```python
from build123d import *

# Parameters (mm, degrees)
F0_R     = 1.5875
F0_W     = 0.381
F0_H     = 9.906
F1_DEPTH = 127
F2_W     = 0.381
F2_H     = 9.906
F3_DEPTH = 127
F7_DEPTH = 127
F5_W     = 1.27
F5_H     = 3.81
F8_DEPTH = 3.175


with BuildPart() as f1:
    # F0 (on Front) → F1 (new body, symmetric)
    with BuildSketch(Plane.XZ):
        Polygon((-8.89, 2.921), (-8.89, -2.921), (-1.4605, -2.921), (-1.0795, -2.921), (1.0795, -2.921), (1.4605, -2.921), (8.89, -2.921), (8.89, 2.921), (3.048, 2.921), (3.048, 9.271), (-3.048, 9.271), (-3.048, 2.921), align=None)
        with Locations((-5.715, 0)):
            Circle(F0_R, mode=Mode.SUBTRACT)
        with Locations((5.715, 0)):
            Circle(F0_R, mode=Mode.SUBTRACT)
        with Locations((-1.27, -7.874)):
            Rectangle(F0_W, F0_H)
        with Locations((1.27, -7.874)):
            Rectangle(F0_W, F0_H)
    extrude(amount=F1_DEPTH, both=True)

    # F2 (on Right) → F3 (intersect, symmetric)
    with BuildSketch(Plane.YZ):
        Polygon((-8.89, 9.271), (-12.954, 9.271), (-12.954, -2.921), (-11.7475, -2.921), (-11.3665, -2.921), (-1.5875, -2.921), (-1.2065, -2.921), (0, -2.921), (0, 9.271), (-3.81, 9.271), (-3.81, 0.1778), (-8.89, 0.1778), align=None)
        with Locations((-1.397, -7.874)):
            Rectangle(F2_W, F2_H)
        with Locations((-11.557, -7.874)):
            Rectangle(F2_W, F2_H)
    extrude(amount=F3_DEPTH, both=True, mode=Mode.INTERSECT)

    # F6 (on Top) → F7 (intersect, symmetric)
    with BuildSketch(Plane.XY):
        Polygon((8.89, 0), (-8.89, 0), (-8.89, -1.905), (-3.048, -1.905), (-3.048, -12.954), (3.048, -12.954), (3.048, -1.905), (8.89, -1.905), align=None)
    extrude(amount=F7_DEPTH, both=True, mode=Mode.INTERSECT)

    # F5 (on plane+point) → F8 (cut, symmetric)
    with BuildSketch(Plane.XZ.offset(6.477)):
        with Locations((0, 7.366)):
            Rectangle(F5_W, F5_H)
    extrude(amount=F8_DEPTH, both=True, mode=Mode.SUBTRACT)


solid = f1.part
```
Could you check a few things on this model? Use its own coordinates, in mm. A direction names the side the tool comes from. Coordinates: 2 decimals unless noted, no trailing zeros. Write each loop counter-clockwise with the first axis right and the second up, starting at its lowest first coordinate (ties: lowest second). Pieces come first, ordered by that corner, then holes. Notation, with made-up numbers: (17, -21.75) -> (31, -21.75) arc R21 ccw to (31, 0.25) -> close; hole circle Ø7 at (12.5, -40). An arc over 180 degrees is marked (long way). One line per question, with ' | ' between items. Start each with the question number.
1. Thinking about a two-plate mould opening in Y: for faces 1 (the face through (0, -6, 0.178)), 2 (the face through (0, -11, 9.271)), 3 (the face through (-7.31, -1.905, 0.69)), which applies, pulls with the +Y half, pulls with the -Y half, needs draft (parallel to the pull), parting line crosses it, or undercut?
2. If we section it at B-B (x = -6.5): Please give me the cut outline in (y, z) (3 decimals), and give its area (3 significant figures).
3. Please list where these lines run through material, in increasing order: line 1 along X through (y, z) = (-0.45, 0); line 2 along Y through (x, z) = (1, 6.5); line 3 along Z through (x, y) = (2.75, -11.5).
4. If we section it at C-C (z = -9.75): Please give me the cut outline in (x, y), and give its area (3 significant figures).
5. For faces 4 (the face through (0, -3.81, 5)), 5 (the face through (-6, -1, 2.921)), 6 (the face through (6, -1, 2.921)), 7 (the face through (0, -3.302, 7)), which set-ups out of +Z, -Z, +X, -X, +Y, -Y let a thin tool reach every point of the face, with its end or its side?
6. If we section it at D-D (y = -8): Please give me the cut outline in (x, z), and give its area (3 significant figures).
7. If we section it at A-A (z = 7): Please give me the cut outline in (x, y) (3 decimals).
8. Will these pins go through, and if not, where does the flat tip stop? P1, Ø2.5, axis at x = 0.5, y = -5.5, coming from the +Z side; P2, Ø4.5, axis at x = 7, z = 0, coming from the -Y side (3 decimals); P3, Ø0.8, axis at y = -9.5, z = 7.5, coming from the -X side.
Return value:
1) face 1: undercut | face 2: needs draft | face 3: pulls with the -Y half
2) outline: (-1.905, -2.921) -> (0, -2.921) -> (0, -1.38) -> (-1.905, -1.38) -> close; (-1.905, 1.38) -> (0, 1.38) -> (0, 2.921) -> (-1.905, 2.921) -> close | area: 5.87 mm²
3) line 1: x = -8.89 to -7.3, -4.13 to 4.13, 7.3 to 8.89 | line 2: y = -12.95 to -8.89, -3.81 to 0 | line 3: z = -2.92 to 9.27
4) outline: (-1.46, -11.75) -> (-1.08, -11.75) -> (-1.08, -11.37) -> (-1.46, -11.37) -> close; (-1.46, -1.59) -> (-1.08, -1.59) -> (-1.08, -1.21) -> (-1.46, -1.21) -> close; (1.08, -11.75) -> (1.46, -11.75) -> (1.46, -11.37) -> (1.08, -11.37) -> close; (1.08, -1.59) -> (1.46, -1.59) -> (1.46, -1.21) -> (1.08, -1.21) -> close | area: 0.581 mm²
5) face 4: +Z, +X, -X | face 5: +Z, -X, +Y, -Y | face 6: +Z, +X, +Y, -Y | face 7: +Z
6) outline: (-3.05, -2.92) -> (3.05, -2.92) -> (3.05, 0.18) -> (-3.05, 0.18) -> close | area: 18.9 mm²
7) outline: (-3.048, -12.954) -> (3.048, -12.954) -> (3.048, -8.89) -> (0.635, -8.89) -> (0.635, -9.652) -> (-0.635, -9.652) -> (-0.635, -8.89) -> (-3.048, -8.89) -> close; (-3.048, -3.81) -> (-0.635, -3.81) -> (-0.635, -3.302) -> (0.635, -3.302) -> (0.635, -3.81) -> (3.048, -3.81) -> (3.048, 0) -> (-3.048, 0) -> close
8) P1: stops at z = 0.18 | P2: stops at y = -1.905 | P3: stops at x = -3.05
